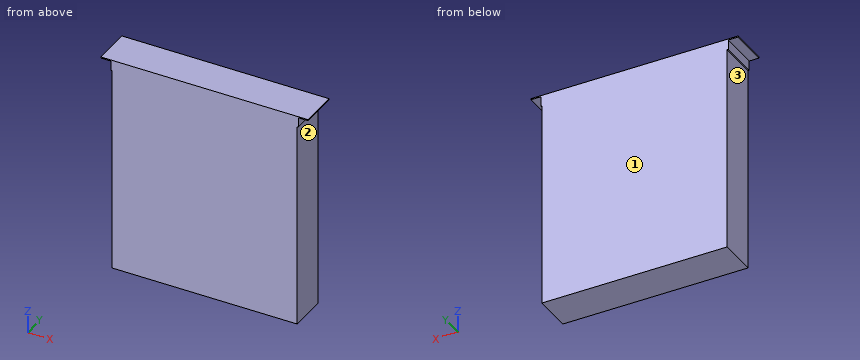
Autodesk Inventor part; units mm, degrees
ref_plane "YZ Plane" through (0, 0, 0) normal (1, 0, 0) x (0, 1, 0)
ref_plane "XZ Plane" through (0, 0, 0) normal (0, 1, 0) x (-1, 0, 0)
ref_plane "XY Plane" through (0, 0, 0) normal (0, 0, 1) x (1, 0, 0)
sketch "Sketch2" plane through (0, 0, 0) normal (0, 1, 0) x (-1, 0, 0)
  line L0 (215.9, 254) -> (-215.9, 254)
  line L1 (-215.9, 254) -> (-215.9, -254)
  line L2 (-215.9, -254) -> (215.9, -254)
  line L3 (215.9, -254) -> (215.9, 254)
  line L4 (215.9, 254) -> (-215.9, -254) construction
  line L5 (-215.9, 254) -> (215.9, -254) construction
  point P0 (0, 0)
  point P1 (0, -254)
  dimension "d6" = 431.8
  dimension "d7" = 508
extrude "Extrusion3" add sketch "Sketch2" along normal blind 88.9
ref_plane "Work Plane3" through (0, 88.9, 254) normal (1, 0, 0) x (0, 1, 0)
sketch "Sketch4" plane through (0, 88.9, 0) normal (0, 1, 0) x (1, 0, 0)
  line L0 (-215.9, -254) -> (215.9, -254)
  line L1 (215.9, -228.6) -> (215.9, -254)
  line L2 (215.9, -254) -> (241.3, -254)
  line L3 (241.3, -251.3584) -> (218.5416, -251.3584)
  line L4 (218.5416, -251.3584) -> (218.5416, -228.6)
  line L5 (215.9, -228.6) -> (218.5416, -228.6)
  line L6 (215.9, -254) -> (215.9, 254)
  line L7 (241.3, -254) -> (241.3, -251.3584)
  point P0 (0, 0)
  dimension "d13" = 25.4
  dimension "d14" = 25.4
  dimension "d15" = 2.6416
extrude "Extrusion5" add sketch "Sketch4" against normal blind 88.9
mirror "Mirror1" about plane through (0, 88.9, 254) normal (1, 0, 0) of "Extrusion5"
equation "\"BendRadius\" = Thickness"
equation "\"BendReliefWidth\" = Thickness"
equation "\"BendReliefDepth\" = 0.5 * Thickness"
equation "\"CornerReliefSize\" = 4 * Thickness"
equation "\"MinimumRemnant\" = 2 * Thickness"
equation "\"TransitionRadius\" = BendRadius"
equation "\"JacobiRadiusSize\" = Thickness"
equation "\"GapSize\" = Thickness"
properties part number "acPower"
The listing builds one solid part. Answer for the finished solid, in the listing's coordinates (mm). Face numbers are marked on the shaded views. A direction names the side the tool comes from. Give positions to 0.01 mm unless a question says otherwise; leave off trailing zeros. Write each loop counter-clockwise with the first axis right and the second up, starting at its lowest first coordinate (ties: lowest second). Pieces come first, ordered by that corner, then holes. Notation, with made-up numbers: (-37.5, 80.5) - (-8.5, 80.5) arc R33 ccw to (-8.5, 118.5) - close; hole circle Ø4 at (-32.5, 45). An arc over 180 degrees is marked (long way). Use a Markdown table: item, result.
1. Each of these flat-tipped pins is pushed along its axis until it touches: P1, Ø10, axis at y = 67, z = -165.5, coming from the -X side; P2, Ø3, axis at x = -218, y = 23.5, coming from the -Z side; P3, Ø18, axis at x = -232.5, y = 39.5, coming from the -Z side; P4, Ø18, axis at y = 56.5, z = 245.5, coming from the -X side. Where does it stop, or does it pass through?
Values follow:
| item | result |
|---|---|
| P1 | stops at x = -215.9 |
| P2 | stops at z = 228.6 |
| P3 | stops at z = 251.36 |
| P4 | stops at x = -241.3 |
2. A tool of negligible diameter and unlimited length cuts with its end or side. For the marked faces 1, 2 and 3, from which of +Z, -Z, +X, -X, +Y, -Y can it reach the whole face along a straight path? Write none if from no direction.
Values follow:
| item | result |
|---|---|
| face 1 | +Z, -Z, +X, -X, +Y |
| face 2 | -Z, +X, +Y, -Y |
| face 3 | -Z, -X, +Y, -Y |
3. Section A-A on y = 59 is taken. Write down the section's boundary in (x, z), plus the area to 3 significant figures.
Values follow:
| item | result |
|---|---|
| outline | (-241.3, 251.36) - (-218.54, 251.36) - (-218.54, 228.6) - (-215.9, 228.6) - (-215.9, -254) - (215.9, -254) - (215.9, 228.6) - (218.54, 228.6) - (218.54, 251.36) - (241.3, 251.36) - (241.3, 254) - (-241.3, 254) - close |
| area | 220,000 mm² |
4. Section B-B on z = 220 is taken. Write down the section's boundary in (x, y), plus the area to 3 significant figures.
Values follow:
| item | result |
|---|---|
| outline | (-215.9, 0) - (215.9, 0) - (215.9, 88.9) - (-215.9, 88.9) - close |
| area | 38,400 mm² |
5. Find the intervals of material crossed by probe 1 along X at (y, z) = (79.5, 31.5); probe 2 along X at (y, z) = (74, 229), in increasing order. Write a range as from..to.
Values follow:
| item | result |
|---|---|
| probe 1 | x = -215.9..215.9 |
| probe 2 | x = -218.54..218.54 |
